```python
from build123d import *

# Parameters (mm, degrees)
SKETCH1_R           = 4
BOSS_EXTRUDE1_DEPTH = 12
CUT_EXTRUDE1_START  = -11
SKETCH2_R           = 4
SKETCH2_R_2         = 3.175
CUT_EXTRUDE1_DEPTH  = 11
SKETCH5_R           = 1.8
CUT_EXTRUDE2_DEPTH  = 14.266499161
SKETCH6_R           = 2.8
CUT_EXTRUDE3_DEPTH  = 4.5


with BuildPart() as part:
    # Sketch1 → Boss-Extrude1 (new body)
    with BuildSketch(Plane.XY):
        Circle(SKETCH1_R)
    extrude(amount=BOSS_EXTRUDE1_DEPTH)

    # Sketch2 → Cut-Extrude1 (cut)
    with BuildSketch(Plane.XY.offset(12).offset(CUT_EXTRUDE1_START)):
        Circle(SKETCH2_R)
        Circle(SKETCH2_R_2, mode=Mode.SUBTRACT)
    extrude(amount=CUT_EXTRUDE1_DEPTH, mode=Mode.SUBTRACT)

    # Sketch5 → Cut-Extrude2 (cut, through all)
    with BuildSketch(Plane(origin=(0, 0, 0), x_dir=(-1, 0, 0), z_dir=(0, 0, -1))):
        Circle(SKETCH5_R)
    extrude(amount=-CUT_EXTRUDE2_DEPTH, mode=Mode.SUBTRACT)

    # Sketch6 → Cut-Extrude3 (cut)
    with BuildSketch(Plane(origin=(0, 0, 0), x_dir=(-1, 0, 0), z_dir=(0, 0, -1))):
        Circle(SKETCH6_R)
    extrude(amount=-CUT_EXTRUDE3_DEPTH, mode=Mode.SUBTRACT)


solid = part.part
```
Here's how the part is built. I have some questions about the finished solid (model axes, mm). A direction names the side the tool comes from. Give positions to 0.01 mm unless a question says otherwise; leave off trailing zeros. Loops run counter-clockwise (first coordinate to the right, second up) from the corner with the lowest first, then second, coordinate; pieces in that order, holes last. Notation, with made-up numbers: M -8,-20.5 L 5,-20.5 A13 cw 5,-4.5 Z; hole C 70,40.5 d5. An arc over 180 degrees is marked long. Return JSON: item names as keys, results as strings.
Item 1: Please list where these lines run through material, in increasing order: line 1 (Y direction, x = 0, z = 9.5) (3 decimals); line 2 (Z direction, x = -1.5, y = 2); line 3 (Z direction, x = 1.5, y = -3).
A:
{"line 1": "y = -3.175 to -1.8, 1.8 to 3.175", "line 2": "z = 4.5 to 12", "line 3": "z = 0 to 1"}
Item 2: Imagine slicing it at A-A on y = 0. List the corners of the cut face in (x, z) for me (3 decimals), then the cut area to 4 significant figures.
A:
{"outline": "M -4,0 L -2.8,0 L -2.8,4.5 L -1.8,4.5 L -1.8,12 L -3.175,12 L -3.175,1 L -4,1 Z; M 1.8,4.5 L 2.8,4.5 L 2.8,0 L 4,0 L 4,1 L 3.175,1 L 3.175,12 L 1.8,12 Z", "area": "25.65 mm^2"}
Item 3: Imagine slicing it at C-C on z = 9.5. List the corners of the cut face in (x, y) for me (3 decimals), then the cut area to 3 significant figures.
A:
{"outline": "C 0,0 d6.35; hole C 0,0 d3.6", "area": "21.5 mm^2"}
Item 4: Imagine slicing it at D-D on y = -2.5. List the corners of the cut face in (x, z) for me.
A:
{"outline": "M -3.12,0 L -1.26,0 L -1.26,4.5 L 1.26,4.5 L 1.26,0 L 3.12,0 L 3.12,1 L 1.96,1 L 1.96,12 L -1.96,12 L -1.96,1 L -3.12,1 Z"}
Item 5: Thinking about a two-plate mould opening in Y: for faces 4 (the flat face through (-3, 2, 1)), 5 (the cylindrical face through (2.8, 0.1, 2.2)), 6 (the cylindrical face through (-0.867, -3.905, 0.493)), which applies, released by +Y, released by -Y, zero draft, split by the parting line, or undercut?
A:
{"face 4": "zero draft", "face 5": "undercut", "face 6": "split by the parting line"}
Item 6: I'm going to push flat-ended pins straight in: pin 1 Ø2 at (x, z) = (-2, 10.5) entering from -Y; pin 2 Ø1.5 at (x, z) = (-2, 3) entering from +Y; pin 3 Ø1.5 at (x, z) = (3, 1.5) entering from +Y. Where does each tip first touch, or does it pass through?
A:
{"pin 1": "stops at y = -3.01", "pin 2": "stops at y = 2.92", "pin 3": "stops at y = 3.17"}
Item 7: On a 3-axis mill with a long thin cutter (end or side, diameter ignored), from which of +Z, -Z, +X, -X, +Y, -Y can I reach the whole of each face in a straight line? I mean faces 1 (the cylindrical face through (-0.69, -3.1, 6.42)), 2 (the flat face through (1.4, -1.4, 12)), 3 (the flat face through (0, -2, 4.5)). Say none if no direction works.
A:
{"face 1": "+Z", "face 2": "+Z, +X, -X, +Y, -Y", "face 3": "-Z"}
